Can you work these out from the model? Positions are in its coordinate system, mm. A direction names the side the tool comes from. Give positions to 0.01 mm unless a question says otherwise; leave off trailing zeros. Write each loop counter-clockwise with the first axis right and the second up, starting at its lowest first coordinate (ties: lowest second). Pieces come first, ordered by that corner, then holes. Notation, with made-up numbers: (88.5, 16) -> (113.5, 16) arc R22 cw to (113.5, 25) -> close; hole circle Ø10 at (86, 48.25). An arc over 180 degrees is marked (long way). One line per item, written item: value.
from build123d import *

# Parameters (mm, degrees)
ESBO_O2_R                           = 10.7
RESSALTO_EXTRUS_O1_DEPTH            = 4.2
RESSALTO_EXTRUS_O3_DEPTH            = 3
ESBO_O5_W                           = 25
ESBO_O5_H                           = 7.051040728
RESSALTO_EXTRUS_O4_DEPTH            = 11.8
REBAIXO_PARA_SHCS_M2_51_D           = 2.9
REBAIXO_PARA_SHCS_M2_51_CBORE_D     = 5.5
REBAIXO_PARA_SHCS_M2_51_CBORE_DEPTH = 10
NERVURA1_REACH                      = 67.976
ESBO_O10_WALL_W                     = 145.845066172
ESBO_O10_WALL_H                     = 15
CORTE_EXTRUS_O1_REACH               = 68.009
ESBO_O11_W                          = 9
ESBO_O11_H                          = 8
ESBO_O12_R                          = 3.25
CORTE_EXTRUS_O2_DEPTH               = 67.475439137
ESBO_O13_R                          = 4
CORTE_EXTRUS_O3_DEPTH               = 6.2
FILETE1_R                           = 2


with BuildPart() as part:
    # Esboço2 → Ressalto-extrusão1 (new body)
    with BuildSketch(Plane.XY.offset(-1.35)):
        with Locations((-0.474928023, -0.063425095)):
            Circle(ESBO_O2_R)
    extrude(amount=-RESSALTO_EXTRUS_O1_DEPTH)

    # Esboço4 → Ressalto-extrusão3 (add)
    with BuildSketch(Plane(origin=(0, 0, -5.55), x_dir=(-1, 0, 0), z_dir=(0, 0, -1))):
        with BuildLine():
            Line((-12.025071977, -0.063425095), (-12.025071977, 64.120162595))
            Line((-12.025071977, 64.120162595), (12.974928023, 64.120162595))
            Line((12.974928023, 64.120162595), (12.974928023, -0.063425095))
            ThreePointArc((12.974928023, -0.063425095), (0.474928023, -12.563425095), (-12.025071977, -0.063425095))
        make_face()
    extrude(amount=RESSALTO_EXTRUS_O3_DEPTH)

    # Esboço5 → Ressalto-extrusão4 (add)
    with BuildSketch(Plane(origin=(0, 0, -8.55), x_dir=(-1, 0, 0), z_dir=(0, 0, -1))):
        with Locations((0.474928023, 60.594642231)):
            Rectangle(ESBO_O5_W, ESBO_O5_H)
    extrude(amount=-RESSALTO_EXTRUS_O4_DEPTH)

    # Rebaixo para SHCS M2.51 (through all)
    with Locations(Plane(origin=(0, 0, -8.55), x_dir=(-1, 0, 0), z_dir=(0, 0, -1))):
        with Locations((-8.49949915, 61.707782077), (8.5, 61.838275999)):
            CounterBoreHole(REBAIXO_PARA_SHCS_M2_51_D / 2, REBAIXO_PARA_SHCS_M2_51_CBORE_D / 2, REBAIXO_PARA_SHCS_M2_51_CBORE_DEPTH)

    # Esboço10 wall → Nervura1 (add, up to next)
    with BuildSketch(Plane(origin=(0, 53.069121867, -1.15), x_dir=(0, -0.672672793996, -0.739940073396), z_dir=(0, 0.739940073396, -0.672672793996)), mode=Mode.PRIVATE) as nervura1_sk1:
        Rectangle(ESBO_O10_WALL_W, ESBO_O10_WALL_H)
    nervura1_tool1 = extrude(nervura1_sk1.sketch, amount=NERVURA1_REACH, mode=Mode.PRIVATE) - part.part
    add(nervura1_tool1.solids().sort_by_distance((0, 53.069121867, -1.15))[0])

    # Esboço11 → Corte-extrusão1 (cut, up to next)
    with BuildSketch(Plane.XY.offset(-5.55), mode=Mode.PRIVATE) as corte_extrus_o1_sk1:
        with Locations((0, 53.069121867)):
            Rectangle(ESBO_O11_W, ESBO_O11_H)
    corte_extrus_o1_tool1 = extrude(corte_extrus_o1_sk1.sketch, amount=CORTE_EXTRUS_O1_REACH, mode=Mode.PRIVATE) & part.part
    add(corte_extrus_o1_tool1.solids().sort_by_distance((0, 53.069122, -5.55))[0], mode=Mode.SUBTRACT)

    # Esboço12 → Corte-extrusão2 (cut, through all)
    with BuildSketch(Plane(origin=(0, 0, -8.55), x_dir=(-1, 0, 0), z_dir=(0, 0, -1))):
        with Locations((0.474928023, -0.063425095)):
            Circle(ESBO_O12_R)
    extrude(amount=-CORTE_EXTRUS_O2_DEPTH, mode=Mode.SUBTRACT)

    # Esboço13 → Corte-extrusão3 (cut)
    with BuildSketch(Plane(origin=(0, 0, -8.55), x_dir=(-1, 0, 0), z_dir=(0, 0, -1))):
        with Locations((0.474928023, -0.063425095)):
            Circle(ESBO_O13_R)
    extrude(amount=-CORTE_EXTRUS_O3_DEPTH, mode=Mode.SUBTRACT)

    # Filete1
    filete1_edges = [part.edges().sort_by_distance(p)[0] for p in [
        (-11.174928023, -0.063425095, -5.55),
    ]]
    fillet(filete1_edges, radius=FILETE1_R - 0.0001)  # a hair under: the kernel refuses the full size


solid = part.part
1) If we section it at B-B (y = 43): Write out the boundary of the cut face in (x, z), and give its area (3 significant figures).
Answer list:
outline: (-12.97, -8.55) -> (12.03, -8.55) -> (12.03, -5.55) -> (-12.97, -5.55) -> close
area: 75.0 mm^2
2) I need wall thicknesses on L1, parallel to Y at x = 0.75, z = -1.5; L2, parallel to Y at x = -8.5, z = 2.3; L3, parallel to Y at x = 6.75, z = -1.5. Which ranges of each line are inside material? Lowest first, please.
Answer list:
L1: y = -10.69 to -3.07, 2.95 to 10.57, 57.07 to 64.12
L2: y = 57.07 to 60.39, 63.29 to 64.12
L3: y = -7.96 to 7.83, 52.75 to 59.59, 63.83 to 64.12
3) For faces 1 (the face through (1.8, 2.5, -1.35)), 2 (the face through (9.41, -4.16, -2.44)), 3 (the face through (-2.321, -3.612, -5.493)), 4 (the face through (7.5, 55, -3)), 5 (the face through (5.979, 53.125, -1.088)), which set-ups out of +Z, -Z, +X, -X, +Y, -Y let a thin tool reach every point of the face, with its end or its side?
Answer list:
face 1: +Z, +X, -X, -Y
face 2: +Z
face 3: -Z
face 4: +Z, +X
face 5: +Z, +X, -X
4) Will these pins go through, and if not, where does the flat tip stop? pin 1 (7.5 mm diameter, centred on x = -6.5, y = 39, fed in from +Z); pin 2 (2 mm diameter, centred on x = 5, y = -4, fed in from +Z); pin 3 (4 mm diameter, centred on y = 54, z = -1, fed in from -X).
Answer list:
pin 1: stops at z = -5.55
pin 2: stops at z = -1.35
pin 3: stops at x = -7.5
5) If we section it at A-A (z = -7.5): Write out the boundary of the cut face in (x, y).
Answer list:
outline: (-12.97, -0.06) arc R12.5 ccw to (12.03, -0.06) -> (12.03, 64.12) -> (9.82, 64.12) arc R2.75 cw (long way) to (7.18, 64.12) -> (-6.97, 64.12) arc R2.75 cw (long way) to (-10.03, 64.12) -> (-12.97, 64.12) -> close; hole circle Ø8 at (-0.47, -0.06)
